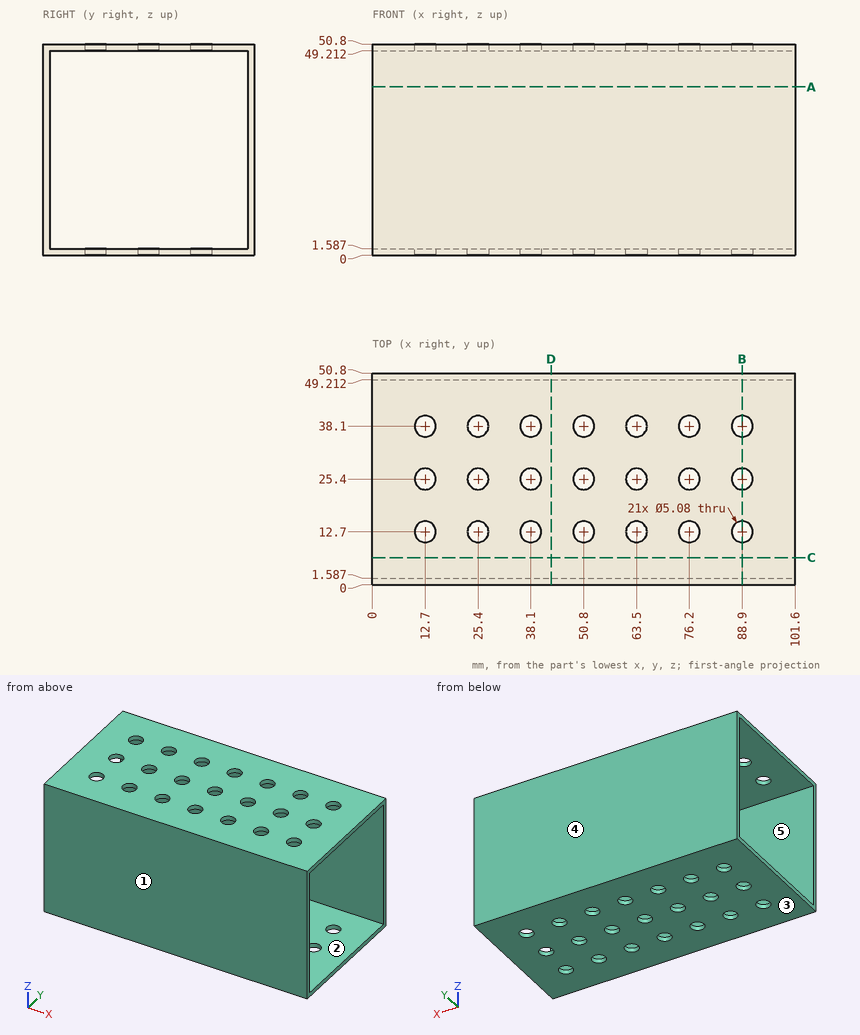
Drawing for the job (mm, zero at the part's lowest x, y, z). A direction names the side the tool comes from. Give positions to 0.01 mm unless a question says otherwise; leave off trailing zeros. Order: outer loops, then holes, each group sorted by start corner. A loop starts at its lowest first (then second) coordinate and runs counter-clockwise, first axis right, second up. Notation, with made-up numbers: (-26, 38) - (14, 38) arc R20 ccw to (14, 64) - close; hole circle Ø2 at (78, 27). An arc over 180 degrees is marked (long way). Use one line per item in the form item = value.
Item 1: Slice it at D-D on x = 43. Give the cut face in (y, z).
Solution:
outline = (0, 0) - (50.8, 0) - (50.8, 50.8) - (0, 50.8) - close; hole (1.59, 1.59) - (49.21, 1.59) - (49.21, 49.21) - (1.59, 49.21) - close
Item 2: Pin check, flat tip, straight feed: pin 1 Ø4.5 at (x, y) = (12.7, 38.1) entering from -Z. Stop position of the tip, or through.
Solution:
pin_1 = through
Item 3: Slice it at B-B on x = 88.9. Count the separate pieces of the cut face and the enclosed holes in it, and give its area (3 significant figures).
Solution:
separate_pieces = 6
enclosed_holes = 0
area = 264 mm2
Item 4: Slice it at A-A on z = 40.5. Give the cut face in (x, y).
Solution:
outline = (0, 0) - (101.6, 0) - (101.6, 1.59) - (0, 1.59) - close; (0, 49.21) - (101.6, 49.21) - (101.6, 50.8) - (0, 50.8) - close
Item 5: Two-plate mould, pull along Y, no slides. Class the marked faces 1, 2 and 3: released by +Y, released by -Y, zero draft, split by the parting line, or undercut.
Solution:
face_1 = released by -Y
face_2 = undercut
face_3 = zero draft
Item 6: Probe probe 1 along Y at (x, z) = (37, 11). List the from-to ranges inside material, lowest first. Write a range as from..to.
Solution:
probe_1 = 0..1.59, 49.21..50.8
Item 7: Which spindle directions (+Z, -Z, +X, -X, +Y, -Y) get a long thin tool onto all of the face, cutting with end or side? Do the marked faces 4 and 5. Say none if no direction does.
Solution:
face_4 = +Z, -Z, +X, -X, +Y
face_5 = +X, -X
